The listing builds one solid part. Answer for the finished solid, in the listing's coordinates (mm). A direction names the side the tool comes from. Coordinates: 2 decimals unless noted, no trailing zeros. Order: outer loops, then holes, each group sorted by start corner. A loop starts at its lowest first (then second) coordinate and runs counter-clockwise, first axis right, second up. Notation, with made-up numbers: (86.25, 52) -> (133.25, 52) arc R38 cw to (133.25, 91) -> close; hole circle Ø9 at (-21, 74). An arc over 180 degrees is marked (long way). Return JSON: item names as keys, results as strings.
from build123d import *

# Parameters (mm, degrees)
ESBO_O1_R                = 1.2
RESSALTO_EXTRUS_O1_DEPTH = 6.3
ESBO_O2_W                = 1.65
ESBO_O2_H                = 3.9
CORTE_EXTRUS_O1_DEPTH    = 21
ESBO_O3_W                = 1.15
ESBO_O3_H                = 6.194421291
CORTE_EXTRUS_O2_DEPTH    = 23.405356502


with BuildPart() as part:
    # Esboço1 → Ressalto-extrusão1 (new body)
    with BuildSketch(Plane.XY):
        Polygon((1.7, -5), (8.2, -5), (8.2, -8.9), (8.6, -8.9), (8.6, -5), (10, -5), (10, 5), (-6.8, 5), (-6.8, 5.642515202), (15.405356502, 11), (15.358448491, 11.194421291), (-7, 5.8), (-7, 5), (-10, 5), (-10, -5), (-7.35, -5), (-7.35, -8.9), (-6.95, -8.9), (-6.95, -5), (1.3, -5), (1.3, -8.9), (1.7, -8.9), align=None)
        with Locations((-4.7, -2.7)):
            Circle(ESBO_O1_R, mode=Mode.SUBTRACT)
        with Locations((4.7, -2.7)):
            Circle(ESBO_O1_R, mode=Mode.SUBTRACT)
    extrude(amount=RESSALTO_EXTRUS_O1_DEPTH)

    # Esboço2 → Corte-extrusão1 (cut, through all)
    with BuildSketch(Plane(origin=(10, 0, 0), x_dir=(0, 0, -1), z_dir=(1, 0, 0))):
        with Locations((-0.825, -6.95)):
            Rectangle(ESBO_O2_W, ESBO_O2_H)
        with Locations((-5.475, -6.95)):
            Rectangle(ESBO_O2_W, ESBO_O2_H)
    extrude(amount=-CORTE_EXTRUS_O1_DEPTH, mode=Mode.SUBTRACT)

    # Esboço3 → Corte-extrusão2 (cut, through all)
    with BuildSketch(Plane.ZY.offset(7)):
        with Locations((0.575, 8.097210646)):
            Rectangle(ESBO_O3_W, ESBO_O3_H)
        with Locations((5.725, 8.097210646)):
            Rectangle(ESBO_O3_W, ESBO_O3_H)
    extrude(amount=-CORTE_EXTRUS_O2_DEPTH, mode=Mode.SUBTRACT)


solid = part.part
1. The part is cut by section A-A on y = -6.5. Give the vertices of the cut face in (x, z), and give its area (3 significant figures).
Answer block:
{"outline": "(-7.35, 1.65) -> (-6.95, 1.65) -> (-6.95, 4.65) -> (-7.35, 4.65) -> close; (1.3, 1.65) -> (1.7, 1.65) -> (1.7, 4.65) -> (1.3, 4.65) -> close; (8.2, 1.65) -> (8.6, 1.65) -> (8.6, 4.65) -> (8.2, 4.65) -> close", "area": "3.60 mm2"}
2. The part is cut by section B-B on z = 0.5. Give the vertices of the cut face in (x, y).
Answer block:
{"outline": "(-10, -5) -> (10, -5) -> (10, 5) -> (-10, 5) -> close; hole circle Ø2.4 at (-4.7, -2.7); hole circle Ø2.4 at (4.7, -2.7)"}
3. Each of these flat-tipped pins is pushed along its axis until it touches: pin 1 Ø0.9 at (y, z) = (-6, 3) entering from -X; pin 2 Ø2 at (x, z) = (-5.5, 1.5) entering from -Y; pin 3 Ø1.9 at (y, z) = (-2, 2) entering from +X. Where does it stop, or does it pass through?
Answer block:
{"pin 1": "stops at x = -7.35", "pin 2": "stops at y = -5", "pin 3": "stops at x = 10"}
4. Determine the mould class of faces 6 (the face through (0, 5, 3)), 7 (the face through (10, 0, 3)), 8 (the face through (4.336, 8.535, 3.122)) for opening direction Y: pulls with the +Y half, pulls with the -Y half, needs draft (parallel to the pull), parting line crosses it, or undercut.
Answer block:
{"face 6": "undercut", "face 7": "needs draft", "face 8": "pulls with the +Y half"}
5. Consider line 1 (X direction, y = -6.5, z = 3); line 2 (X direction, y = -2.5, z = 0.75); line 3 (Y direction, x = -4.7, z = 1.75). Determine where each line is inside the solid, lowest interval first. Write a range as from..to.
Answer block:
{"line 1": "x = -7.35..-6.95, 1.3..1.7, 8.2..8.6", "line 2": "x = -10..-5.88, -3.52..3.52, 5.88..10", "line 3": "y = -5..-3.9, -1.5..5, 6.15..6.35"}
6. The part is cut by section C-C on x = -2.75. Give the vertices of the cut face in (y, z).
Answer block:
{"outline": "(-5, 0) -> (5, 0) -> (5, 6.3) -> (-5, 6.3) -> close; (6.62, 1.15) -> (6.83, 1.15) -> (6.83, 5.15) -> (6.62, 5.15) -> close"}
7. The part is cut by section D-D on x = 4.7. Give the vertices of the cut face in (y, z), and give its area (3 significant figures).
Answer block:
{"outline": "(-5, 0) -> (-3.9, 0) -> (-3.9, 6.3) -> (-5, 6.3) -> close; (-1.5, 0) -> (5, 0) -> (5, 6.3) -> (-1.5, 6.3) -> close; (8.42, 1.15) -> (8.62, 1.15) -> (8.62, 5.15) -> (8.42, 5.15) -> close", "area": "48.7 mm2"}
8. For faces 1 (the face through (-7.35, -7, 3)), 2 (the face through (8.6, -7, 3)), 3 (the face through (-10, 0, 3)), 4 (the face through (1.7, -7, 3)), 5 (the face through (4.147, 8.284, 3.122)), determine the directions among +Z, -Z, +X, -X, +Y, -Y from which every point of the face is accessible in a straight line to the end or side of a thin tool.
Answer block:
{"face 1": "+Z, -Z, -X, -Y", "face 2": "+Z, -Z, +X, -Y", "face 3": "+Z, -Z, -X, +Y, -Y", "face 4": "+Z, -Z, -Y", "face 5": "+Z, -Z, +X"}
